```python
from build123d import *

# Parameters (mm, degrees)
SKETCH1_R           = 74.45
SKETCH1_R_2         = 2.25
SKETCH1_R_3         = 17
BOSS_EXTRUDE1_DEPTH = 2
SKETCH2_R           = 19
SKETCH2_R_2         = 17
BOSS_EXTRUDE2_DEPTH = 10
SKETCH3_R           = 74.45
SKETCH3_R_2         = 72.45
BOSS_EXTRUDE3_DEPTH = 3


with BuildPart() as part:
    # Sketch1 → Boss-Extrude1 (new body)
    with BuildSketch(Plane(origin=(0, 0, 0), x_dir=(1, 0, 0), z_dir=(0, 1, 0))):
        with Locations(Location((0, 0, 0), (0, 0, 270))):
            Circle(SKETCH1_R)
        with Locations(Location((68, 0, 0), (0, 0, 270))):
            Circle(SKETCH1_R_2, mode=Mode.SUBTRACT)
        with Locations(Location((0, -68, 0), (0, 0, 270))):
            Circle(SKETCH1_R_2, mode=Mode.SUBTRACT)
        with Locations(Location((-68, 0, 0), (0, 0, 270))):
            Circle(SKETCH1_R_2, mode=Mode.SUBTRACT)
        with Locations(Location((0, 68, 0), (0, 0, 270))):
            Circle(SKETCH1_R_2, mode=Mode.SUBTRACT)
        with Locations(Location((0, 0, 0), (0, 0, 270))):
            Circle(SKETCH1_R_3, mode=Mode.SUBTRACT)
    extrude(amount=BOSS_EXTRUDE1_DEPTH)

    # Sketch2 → Boss-Extrude2 (add)
    with BuildSketch(Plane(origin=(0, 2, 0), x_dir=(1, 0, 0), z_dir=(0, 1, 0))):
        with Locations(Location((0, 0, 0), (0, 0, 270))):
            Circle(SKETCH2_R)
        with Locations(Location((0, 0, 0), (0, 0, 270))):
            Circle(SKETCH2_R_2, mode=Mode.SUBTRACT)
    extrude(amount=BOSS_EXTRUDE2_DEPTH)

    # Sketch3 → Boss-Extrude3 (add)
    with BuildSketch(Plane(origin=(0, 2, 0), x_dir=(1, 0, 0), z_dir=(0, 1, 0))):
        with Locations(Location((0, 0, 0), (0, 0, 270))):
            Circle(SKETCH3_R)
        with Locations(Location((0, 0, 0), (0, 0, 270))):
            Circle(SKETCH3_R_2, mode=Mode.SUBTRACT)
    extrude(amount=BOSS_EXTRUDE3_DEPTH)


solid = part.part
```
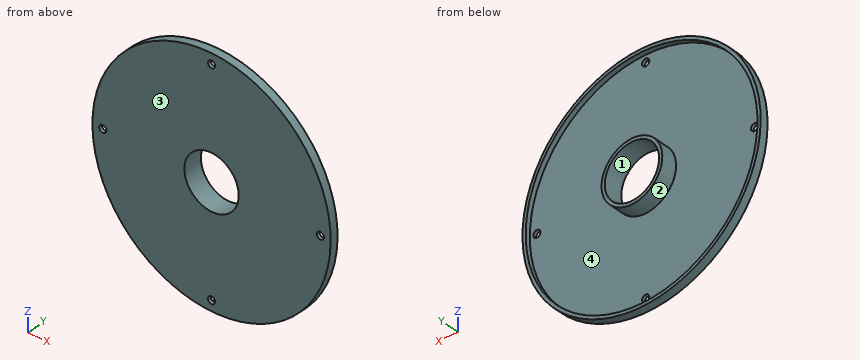
Input: part model. Units: mm. Frame: model coordinates. Face numbers are marked on the shaded views. A direction names the side the tool comes from. Give positions to 0.01 mm unless a question says otherwise; leave off trailing zeros. Write each loop counter-clockwise with the first axis right and the second up, starting at its lowest first coordinate (ties: lowest second). Pieces come first, ordered by that corner, then holes. Notation, with made-up numbers: (55, 13) - (96, 13) arc R15 cw to (96, 28) - close; hole circle Ø5 at (27, -19.75). An arc over 180 degrees is marked (long way). Write item = value, one per line. Start each with the question number.
1. Ray query, L1, parallel to X at y = 8.5, z = 0; L2, parallel to Y at x = -18.5, z = 68; L3, parallel to Z at x = -2.5, y = 1.5. Return the intervals inside material, ascending.
2. Section query B-B, the plane z = 0. Output: boundary loops of the cut face in (x, y).
3. Section query D-D, the plane x = -68. Output: boundary loops of the cut face in (y, z).
4. Access query for the marked faces 1 and 2. Directions: +Z, -Z, +X, -X, +Y, -Y. A direction counts if a zero-diameter tool reaches every point of the face in a straight line with its end or side. Return the directions, or none.
5. Section query C-C, the plane z = 68. Output: boundary loops of the cut face in (x, y).
6. First-contact query: pin 1 Ø6 at (x, z) = (-68, 0) entering from +Y; pin 2 Ø5 at (x, z) = (0, -68) entering from -Y; pin 3 Ø1.5 at (x, y) = (17, 7.5) entering from +Z; pin 4 Ø5 at (y, z) = (9.5, 20) entering from +X. Flat tips, straight axial feed; report the tip coordinate or a pass-through.
7. Mould query, pull axis X, two halves, no side actions, for the marked faces 3 and 4. Classes: released by +X, released by -X, zero draft, split by the parting line, or undercut.
8. Section query A-A, the plane x = 0. Output: boundary loops of the cut face in (y, z), then the cut area to 3 significant figures.
Check sheet entries:
q1.L1 = -19 to -17, 17 to 19
q1.L2 = 0 to 2
q1.L3 = -74.41 to -16.82, 16.82 to 74.41
q2.outline = (-74.45, 0) - (-70.25, 0) - (-70.25, 2) - (-72.45, 2) - (-72.45, 5) - (-74.45, 5) - close; (-65.75, 0) - (-17, 0) - (-17, 12) - (-19, 12) - (-19, 2) - (-65.75, 2) - close; (17, 0) - (65.75, 0) - (65.75, 2) - (19, 2) - (19, 12) - (17, 12) - close; (70.25, 0) - (74.45, 0) - (74.45, 5) - (72.45, 5) - (72.45, 2) - (70.25, 2) - close
q3.outline = (0, -30.31) - (5, -30.31) - (5, -25) - (2, -25) - (2, -2.25) - (0, -2.25) - close; (0, 2.25) - (2, 2.25) - (2, 25) - (5, 25) - (5, 30.31) - (0, 30.31) - close
q4.face_1 = +Y, -Y
q4.face_2 = +Y
q5.outline = (-30.31, 0) - (-2.25, 0) - (-2.25, 2) - (-25, 2) - (-25, 5) - (-30.31, 5) - close; (2.25, 0) - (30.31, 0) - (30.31, 5) - (25, 5) - (25, 2) - (2.25, 2) - close
q6.pin_1 = 2
q6.pin_2 = 0
q6.pin_3 = 9.85
q6.pin_4 = 7.4
q7.face_3 = zero draft
q7.face_4 = undercut
q8.outline = (0, -74.45) - (5, -74.45) - (5, -72.45) - (2, -72.45) - (2, -70.25) - (0, -70.25) - close; (0, -65.75) - (2, -65.75) - (2, -19) - (12, -19) - (12, -17) - (0, -17) - close; (0, 17) - (12, 17) - (12, 19) - (2, 19) - (2, 65.75) - (0, 65.75) - close; (0, 70.25) - (2, 70.25) - (2, 72.45) - (5, 72.45) - (5, 74.45) - (0, 74.45) - close
q8.area = 264 mm2
